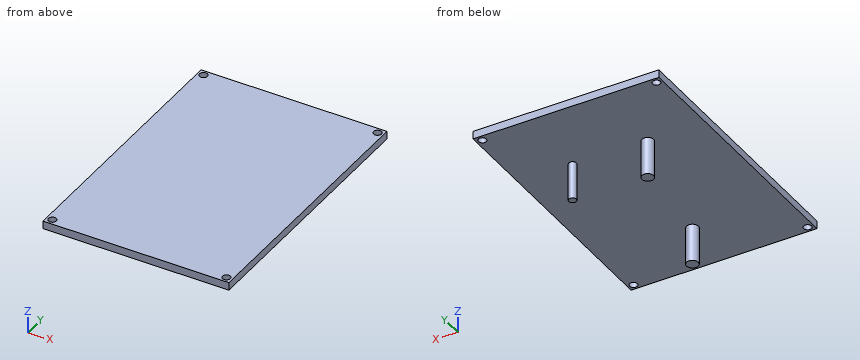
```python
from build123d import *

# Parameters (mm, degrees)
SKETCH1_W           = 70.681980515
SKETCH1_H           = 102.181980515
SKETCH1_R           = 1.5
BOSS_EXTRUDE2_DEPTH = 3
SKETCH1_27_R        = 2.236067977
SKETCH1_27_R_2      = 1.414213562
BOSS_EXTRUDE3_DEPTH = 14.35


with BuildPart() as part:
    # Sketch1 → Boss-Extrude2 (new body)
    with BuildSketch(Plane.XY):
        with Locations((35.340990258, 51.090990258)):
            Rectangle(SKETCH1_W, SKETCH1_H)
        with Locations((68.431980515, 2.25)):
            Circle(SKETCH1_R, mode=Mode.SUBTRACT)
        with Locations((2.25, 99.931980515)):
            Circle(SKETCH1_R, mode=Mode.SUBTRACT)
        with Locations((68.431980515, 99.931980515)):
            Circle(SKETCH1_R, mode=Mode.SUBTRACT)
        with Locations((2.25, 2.25)):
            Circle(SKETCH1_R, mode=Mode.SUBTRACT)
    extrude(amount=BOSS_EXTRUDE2_DEPTH)

    # Sketch1<27> → Boss-Extrude3 (add)
    with BuildSketch(Plane.XY):
        with Locations((35, 21)):
            Circle(SKETCH1_27_R)
        with Locations((50, 73)):
            Circle(SKETCH1_27_R_2)
        with Locations((22, 72)):
            Circle(SKETCH1_27_R)
    extrude(amount=-BOSS_EXTRUDE3_DEPTH)


solid = part.part
```
Input: part model. Units: mm. Frame: model coordinates. Give positions to 0.01 mm unless a question says otherwise; leave off trailing zeros. Write each loop counter-clockwise with the first axis right and the second up, starting at its lowest first coordinate (ties: lowest second). Pieces come first, ordered by that corner, then holes. Notation, with made-up numbers: (-20.75, 49) - (37.25, 49) arc R10 ccw to (37.25, 61) - close; hole circle Ø6 at (77.5, -12.5). An arc over 180 degrees is marked (long way). Write item = value, one per line. Start each with the question number.
1) Pin query (flat end, axial travel): pin 1 (4 mm diameter, centred on x = 68.43, y = 99.93, fed in from -Z); pin 2 (4 mm diameter, centred on x = 2.25, y = 2.25, fed in from +Z); pin 3 (1.5 mm diameter, centred on x = 52.5, z = -11, fed in from -Y). Return the tip coordinate at first contact, or that it passes through.
2) Cut plane D-D (x = 50). Return loops of the section in (y, z).
3) Cut plane B-B (y = 2.25). Return loops of the section in (x, z), and give its area (3 significant figures).
4) Material intervals for L1, parallel to Y at x = 2.25, z = 1.3; L2, parallel to Z at x = 30, y = 93; L3, parallel to Y at x = 37, z = -10.25, sorted ascending. Write a range as [from, to].
5) Cut plane A-A (x = 2.25). Return loops of the section in (y, z).
6) Cut plane C-C (z = -7.75). Return loops of the section in (x, y).
Answers follow:
q1.pin_1 = 0
q1.pin_2 = 3
q1.pin_3 = through
q2.outline = (0, 0) - (71.59, 0) - (71.59, -14.35) - (74.41, -14.35) - (74.41, 0) - (102.18, 0) - (102.18, 3) - (0, 3) - close
q3.outline = (0, 0) - (0.75, 0) - (0.75, 3) - (0, 3) - close; (3.75, 0) - (66.93, 0) - (66.93, 3) - (3.75, 3) - close; (69.93, 0) - (70.68, 0) - (70.68, 3) - (69.93, 3) - close
q3.area = 194 mm^2
q4.L1 = [0, 0.75], [3.75, 98.43], [101.43, 102.18]
q4.L2 = [0, 3]
q4.L3 = [20, 22]
q5.outline = (0, 0) - (0.75, 0) - (0.75, 3) - (0, 3) - close; (3.75, 0) - (98.43, 0) - (98.43, 3) - (3.75, 3) - close; (101.43, 0) - (102.18, 0) - (102.18, 3) - (101.43, 3) - close
q6.outline = circle Ø4.47 at (22, 72); circle Ø4.47 at (35, 21); circle Ø2.83 at (50, 73)
